```python
from build123d import *

# Parameters (mm, degrees)
EXTRUDE_1_DEPTH = 67
SKETCH_3_W      = 1
SKETCH_3_H      = 7


with BuildPart() as part:
    # Эскиз1 → Бобышка-Вытянуть1 (new body)
    with BuildSketch(Plane(origin=(0, 0, 0), x_dir=(0, 0, -1), z_dir=(1, 0, 0))):
        Polygon((-6, 0.35), (-0.35, 0.35), (-0.35, 6), (0.35, 6), (0.35, 0.35), (6, 0.35), (6, -0.35), (0.35, -0.35), (0.35, -6), (-0.35, -6), (-0.35, -0.35), (-6, -0.35), align=None)
    extrude(amount=EXTRUDE_1_DEPTH)

    # Эскиз3 → Повернуть1 (revolve)
    with BuildSketch(Plane.XY):
        Polygon((74.75277675, 0), (71, 6.5), (67, 6.5), (67, 0), align=None)
        with Locations((-0.5, 3.5)):
            Rectangle(SKETCH_3_W, SKETCH_3_H)
    revolve(axis=Axis((0, 0, 0), (1, 0, 0)))

    # Эскиз4 → Вырез-Повернуть1 (revolve, cut)
    with BuildSketch(Plane.XY):
        with BuildLine():
            Line((0, 6), (0, 3.175))
            Line((0, 3.175), (11.953250745, 3.175))
            add(Edge.make_bspline(
                [(11.953250745, 3.175), (13.82559534, 3.302015048), (23.044496857, 6.133590622), (30.696517759, 12.611861304), (39.780139318, 8.557592838)],
                knots=[0, 0, 0, 0, 0.195436417, 1, 1, 1, 1], degree=3))
            Line((39.780139318, 8.557592838), (39.780139318, 6))
            Line((39.780139318, 6), (41.904336104, 3.875803214))
            Line((41.904336104, 3.875803214), (45.076323965, 7.047791075))
            Line((45.076323965, 7.047791075), (24.996442716, 20.783696601))
            Line((24.996442716, 20.783696601), (10.913533525, 15.605616348))
            Line((10.913533525, 15.605616348), (0, 6))
        make_face()
    revolve(axis=Axis((0, 0, 0), (1, 0, 0)), mode=Mode.SUBTRACT)


solid = part.part
```
CAD build for the part. Positions are in the model's coordinates, mm. A direction names the side the tool comes from. Coordinates: 2 decimals unless noted, no trailing zeros. Write each loop counter-clockwise with the first axis right and the second up, starting at its lowest first coordinate (ties: lowest second). Pieces come first, ordered by that corner, then holes.
(1) Flat gauge pins, fed straight in: pin 1 (3 mm diameter, centred on x = 49.5, y = 2, fed in from +Z); pin 2 (6 mm diameter, centred on x = 35.5, y = 4, fed in from -Z); pin 3 (6 mm diameter, centred on x = 39, z = -3.5, fed in from -Y). Where does each tip first touch, or does it go through?
(2) Cut at B-B, the plane z = 5. Count the separate pieces of the cut face and the enclosed holes in it, and give its area (3 significant figures).
(3) Drill centre lines: probe 1 along Y at (x, z) = (49, -4.5); probe 2 along Z at (x, y) = (63.5, 0). Where is each one in solid material? Low to high.
(4) Cut at D-D, the plane x = 6.5. List the corners of the cut face in (y, z) (3 decimals).
(5) 3-axis set-ups, long thin cutter, end or side, ignore diameter. For faces 1 (the face through (40, -0.35, -3)), 2 (the face through (33, 3, 0.35)), 3 (the face through (33, 0.35, -3)), 4 (the face through (42.99, -4.96, 0.01)): which of +Z, -Z, +X, -X, +Y, -Y reach the whole face in a straight line?
(6) Two-plate mould, pull along X, no slides. Class faces 5 (the face through (40.86, -0.01, -4.92)), 6 (the face through (-1, 0, 0)), 7 (the face through (-0.493, 6.466, -2.681)): +X half, -X half, draft (parallel to the pull), parting line (faces both ways), or undercut.
(7) Cut at A-A, the plane x = 51. List the corners of the cut face in (y, z).
Geometry says:
1. pin 1: stops at z = 0.35
1. pin 2: stops at z = -0.35
1. pin 3: stops at y = -0.35
2. separate pieces: 3
2. enclosed holes: 0
2. area: 80.1 mm2
3. probe 1: y = -0.35 to 0.35
3. probe 2: z = -6 to 6
4. outline: (-3.156, -0.35) - (-0.35, -0.35) - (-0.35, -3.156) arc R3.175 ccw to (0.35, -3.156) - (0.35, -0.35) - (3.156, -0.35) arc R3.175 ccw to (3.156, 0.35) - (0.35, 0.35) - (0.35, 3.156) arc R3.175 ccw to (-0.35, 3.156) - (-0.35, 0.35) - (-3.156, 0.35) arc R3.175 ccw to start
5. face 1: -Z, -Y
5. face 2: +Z, +Y
5. face 3: -Z, +Y
5. face 4: -Y
6. face 5: undercut
6. face 6: -X half
6. face 7: draft
7. outline: (-6, -0.35) - (-0.35, -0.35) - (-0.35, -6) - (0.35, -6) - (0.35, -0.35) - (6, -0.35) - (6, 0.35) - (0.35, 0.35) - (0.35, 6) - (-0.35, 6) - (-0.35, 0.35) - (-6, 0.35) - close
